Work out the finished part from the listing and answer in its coordinate system (mm). Give positions to 0.01 mm unless a question says otherwise; leave off trailing zeros. Loops run counter-clockwise (first coordinate to the right, second up) from the corner with the lowest first, then second, coordinate; pieces in that order, holes last. Notation, with made-up numbers: (60.5, -26) -> (68.5, -26) arc R24 ccw to (68.5, -13) -> close; hole circle Ø11 at (63.25, 79). An arc over 180 degrees is marked (long way). Answer as CSV lines item,"result". Start each with the question number.
1. Find section A-A, the plane x = 95.3. Give the vertices of the cut face in (y, z).
2. Find the intervals of material crossed by line 1 along Z through (x, y) = (93.5, 2.4); line 2 along Z through (x, y) = (95.3, 1.5); line 3 along X through (y, z) = (1.9, -282), in increasing order.
3. Find section D-D, the plane x = 79. Give the vertices of the cut face in (y, z), and give its area (3 significant figures).
4. Find section C-C, the plane z = -254. Give the vertices of the cut face in (x, y).
5. Find section B-B, the plane y = 1.9. Give the vertices of the cut face in (x, z), and give its area (3 significant figures).
6. Flat-ended cylindrical pins translate along their axes: pin 1 Ø10 at (x, z) = (108.5, -262) entering from -Y; pin 2 Ø1 at (x, y) = (156, 1) entering from -Z. Find the tip coordinate at first contact, or state that the pin passes through.
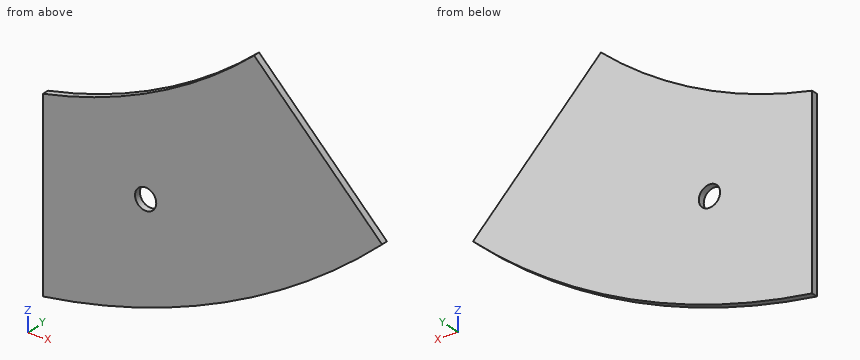
Autodesk Inventor part; units mm, degrees
ref_plane "YZ Plane" through (0, 0, 0) normal (1, 0, 0) x (0, 1, 0)
ref_plane "XZ Plane" through (0, 0, 0) normal (0, 1, 0) x (-1, 0, 0)
ref_plane "XY Plane" through (0, 0, 0) normal (0, 0, 1) x (1, 0, 0)
sketch "Sketch1" plane through (0, 0, 0) normal (0, 1, 0) x (-1, 0, 0)
  circle A0 centre (0, 0) radius 215
  circle A1 centre (0, 0) radius 315
  line L0 (0, 0) -> (0, -315)
  line L1 (0, 0) -> (-222.7386, -222.7386)
  line L2 (-141.0509, -162.2641) -> (-211.8794, -233.0926)
  line L3 (-15, -214.4761) -> (-15, -314.6427)
  circle A2 centre (0, 0) radius 222.5
  circle A3 centre (0, 0) radius 307.5
  line L4 (-47, -311.4739) -> (-47, -209.7999)
  point P0 (-152.028, -152.028)
  point P1 (0, -215)
  point P2 (0, -312.5)
  point P3 (0, -217.5)
  point P4 (-153.7957, -153.7957)
  point P5 (-220.9709, -220.9709)
  point P6 (-210.1096, -231.3228)
  point P7 (-15, -312.1398)
  point P8 (-15, -216.9821)
  point P9 (-142.8229, -164.0361)
  point P10 (-206.5699, -227.7831)
  point P11 (-15, -307.1339)
  point P12 (-15, -221.9938)
  point P13 (-146.3667, -167.5799)
  point P14 (-47, -303.8869)
  point P15 (-47, -217.4793)
  dimension "d2" = 430
  dimension "d3" = 630
  dimension "d4" = 45
  dimension "d5" = 15
  dimension "d6" = 15
  dimension "d11" = 7.5
  dimension "d12" = 7.5
  dimension "d16" = 32
extrude "Extrusion1" add sketch "Sketch1" along normal blind 3 contours A2 L4 A3 L2 | A2 L3 A3 L4
sketch "Sketch4" plane through (0, 0, 0) normal (0, 0, 1) x (1, 0, 0)
  line L0 (15, 0) -> (146.3667, 0)
  line L1 (146.3667, 0) -> (146.3667, 3)
  line L2 (15, 3) -> (146.3667, 3)
  line L3 (15, 0) -> (15, 3)
  line L4 (15, 0) -> (47, 0)
  line L5 (47, 0) -> (47, 3)
  line L6 (47, 3) -> (15, 3)
  line L7 (15, 3) -> (15, 0)
  point P0 (0, 0)
  dimension "d17" = 32
extrude "Extrusion3" cut sketch "Sketch4" against normal up to surface contours L3 L2 L5 L0
sketch "Sketch5" plane through (0, 3, 0) normal (0, 1, 0) x (1, 0, 0)
  line L0 (47, 303.8869) -> (47, 217.4793)
  arc A0 (146.3667, 167.5799) -> (47, 217.4793) centre (0, 0) ccw
  line L1 (146.3667, 167.5799) -> (206.5699, 227.7831)
  arc A1 (206.5699, 227.7831) -> (47, 303.8869) centre (0, 0) ccw
  line L2 (146.3667, 167.5799) -> (206.5699, 227.7831)
  line L3 (47, 217.4793) -> (47, 303.8869)
  circle A2 centre (50, 219.8092) radius 1.75
  circle A3 centre (143.9011, 173.5996) radius 1.75
  circle A4 centre (199.96, 229.6585) radius 1.75
  circle A5 centre (50, 300.4077) radius 1.75
  arc A6 (146.3667, 167.5799) -> (47, 217.4793) centre (0, 0) ccw
  line L4 (99.8507, 198.8368) -> (132.3721, 277.5498) construction
  arc A7 (206.5699, 227.7831) -> (47, 303.8869) centre (0, 0) ccw
  line L5 (116.1114, 238.1933) -> (47, 266.7477) construction
  line L6 (116.1114, 238.1933) -> (187.4893, 208.7025) construction
  line L7 (50, 300.4077) -> (50, 298.6577) construction
  line L8 (50, 300.4077) -> (47, 300.4077) construction
  line L9 (143.9011, 173.5996) -> (148.1437, 169.3569) construction
  line L10 (50, 219.8092) -> (47, 219.8092) construction
  line L11 (199.96, 229.6585) -> (204.2027, 225.4159) construction
  line L12 (50, 216.8092) -> (50, 303.4077) construction
  line L13 (141.7806, 171.4774) -> (202.1185, 231.742) construction
  dimension "d36" = 3.5
  dimension "d37" = 3
  dimension "d40" = 3.5
  dimension "d45" = 6
  dimension "d47" = 3.5
  dimension "d48" = 3.5
  dimension "d49" = 6
  dimension "d51" = 3
  dimension "d53" = 3
  dimension "d54" = 3
  dimension "d55" = 3
  dimension "d56" = 3
extrude "Extrusion4" [suppressed]
sketch "Sketch6" plane through (0, 3, 0) normal (0, 1, 0) x (1, 0, 0)
  line L0 (47, 303.8869) -> (47, 217.4793)
  arc A0 (146.3667, 167.5799) -> (47, 217.4793) centre (0, 0) ccw
  line L1 (146.3667, 167.5799) -> (206.5699, 227.7831)
  arc A1 (206.5699, 227.7831) -> (47, 303.8869) centre (0, 0) ccw
  line L2 (0, 0) -> (132.3721, 277.5498)
  arc A2 (206.5699, 227.7831) -> (47, 303.8869) centre (0, 0) ccw
  arc A3 (146.3667, 167.5799) -> (47, 217.4793) centre (0, 0) ccw
  line L3 (95.7814, 200.8287) -> (132.3721, 277.5498)
  line L4 (114.0768, 239.1892) -> (95.7814, 200.8287)
  line L5 (146.3667, 167.5799) -> (206.5699, 227.7831)
  line L6 (176.4683, 197.6815) -> (47, 260.6831)
  line L7 (47, 217.4793) -> (47, 303.8869)
  circle A4 centre (95.3, 246.0764) radius 5
  point P0 (104.9291, 220.009)
  dimension "d61" = 10
  dimension "d62" = 20
  dimension "d63" = 8
extrude "Extrusion5" cut sketch "Sketch6" against normal blind 10 contours A4
properties part number "Battery Module Third Iteration" material "PLA Plastic"
Resolved:
1,outline,"(0, -292.36) -> (3, -292.36) -> (3, -251.08) -> (0, -251.08) -> close; (0, -241.08) -> (3, -241.08) -> (3, -201.06) -> (0, -201.06) -> close"
2,line 1,"z = -292.94 to -250.74, -241.41 to -201.9"
2,line 2,"z = -292.36 to -251.08, -241.08 to -201.06"
2,line 3,"x = 47 to 122.61"
3,outline,"(0, -297.18) -> (3, -297.18) -> (3, -208) -> (0, -208) -> close"
3,area,"268 mm^2"
4,outline,"(47, 0) -> (173.32, 0) -> (173.32, 3) -> (47, 3) -> close"
5,outline,"(47, -303.89) arc R307.5 ccw to (206.57, -227.78) -> (146.37, -167.58) arc R222.5 cw to (47, -217.48) -> close; hole circle Ø10 at (95.3, -246.08)"
5,area,"12,300 mm^2"
6,pin 1,"stops at y = 0"
6,pin 2,"stops at z = -265.28"
